from build123d import *

# Parameters (mm, degrees)
SKETCH1_R           = 1.75
BOSS_EXTRUDE1_DEPTH = 2.5
CUT_EXTRUDE1_DEPTH  = 0.2
SKETCH5_R           = 3
CUT_EXTRUDE2_DEPTH  = 0.5
CHAMFER2_SIZE       = 1


with BuildPart() as part:
    # Sketch1 → Boss-Extrude1 (new body)
    with BuildSketch(Plane.XY):
        with BuildLine():
            ThreePointArc((-28.95, 27.5), (-33.45, 23), (-28.95, 18.5))
            Line((-28.95, 18.5), (-24.45, 18.5))
            Line((-24.45, 18.5), (-24.45, -18.5))
            Line((-24.45, -18.5), (-28.95, -18.5))
            ThreePointArc((-28.95, -18.5), (-33.45, -23), (-28.95, -27.5))
            Line((-28.95, -27.5), (28.95, -27.5))
            ThreePointArc((28.95, -27.5), (33.45, -23), (28.95, -18.5))
            Line((28.95, -18.5), (24.45, -18.5))
            Line((24.45, -18.5), (24.45, 18.5))
            Line((24.45, 18.5), (28.95, 18.5))
            ThreePointArc((28.95, 18.5), (33.45, 23), (28.95, 27.5))
            Line((28.95, 27.5), (-28.95, 27.5))
        make_face()
        with Locations((-28.95, -23)):
            Circle(SKETCH1_R, mode=Mode.SUBTRACT)
        with Locations((-28.95, 23)):
            Circle(SKETCH1_R, mode=Mode.SUBTRACT)
        with Locations((28.95, 23)):
            Circle(SKETCH1_R, mode=Mode.SUBTRACT)
        with Locations((28.95, -23)):
            Circle(SKETCH1_R, mode=Mode.SUBTRACT)
    extrude(amount=BOSS_EXTRUDE1_DEPTH)

    # Sketch4 → Cut-Extrude1 (cut)
    with BuildSketch(Plane.XY.offset(2.5)):
        with BuildLine():
            Line((-6.923076923, -4.414458023), (-8.846153846, -4.414458023))
            Line((-8.846153846, -4.414458023), (-8.846153846, 2.704933003))
            add(Edge.make_bspline(
                [(-8.846153846, 2.704933003), (-8.933318023, 2.616445103), (-9.106463901, 2.440669737), (-9.383005145, 2.19548654), (-9.670097117, 1.967401521), (-9.970580856, 1.758581072), (-10.280528273, 1.566049869), (-10.603106853, 1.391327059), (-10.935978437, 1.231995104), (-11.166572995, 1.142953291), (-11.282051282, 1.09836249)],
                knots=[0, 0, 0, 0, 0.000372537, 0.00074002, 0.001107934, 0.001471928, 0.001837155, 0.002201986, 0.002572064, 0.002943306, 0.002943306, 0.002943306, 0.002943306], degree=3))
            Line((-11.282051282, 1.09836249), (-11.282051282, 3.021439413))
            add(Edge.make_bspline(
                [(-11.282051282, 3.021439413), (-11.153980048, 3.06946063), (-10.88593692, 3.1699653), (-10.490395403, 3.38374383), (-10.077539391, 3.648423218), (-9.730716774, 3.908012402), (-9.455353873, 4.138807932), (-9.26289614, 4.324331325), (-9.084572984, 4.514316902), (-8.927087219, 4.714896702), (-8.786304768, 4.922015444), (-8.661565378, 5.135334763), (-8.551766041, 5.355528522), (-8.494286856, 5.508866571), (-8.465544872, 5.585541977)],
                knots=[0, 0, 0, 0, 0.000409928, 0.000857948, 0.001345291, 0.001880548, 0.002156279, 0.002422637, 0.002682042, 0.002937331, 0.003186801, 0.003432796, 0.003678268, 0.003923781, 0.003923781, 0.003923781, 0.003923781], degree=3))
            Line((-8.465544872, 5.585541977), (-6.923076923, 5.585541977))
            Line((-6.923076923, 5.585541977), (-6.923076923, -4.414458023))
        make_face()
        with BuildLine():
            Line((2.435897436, -2.4913811), (2.435897436, -4.414458023))
            Line((2.435897436, -4.414458023), (-4.102564103, -4.414458023))
            add(Edge.make_bspline(
                [(-4.102564103, -4.414458023), (-4.080426387, -4.250103198), (-4.036163368, -3.921485704), (-3.899317938, -3.441458257), (-3.716676165, -2.973033485), (-3.518453211, -2.59184942), (-3.321298527, -2.285009365), (-3.142420071, -2.033582253), (-2.929024642, -1.766074598), (-2.684208836, -1.480326872), (-2.409325608, -1.175445832), (-2.102324151, -0.852564961), (-1.761740021, -0.513229981), (-1.522133018, -0.282804832), (-1.398237179, -0.163656741)],
                knots=[0, 0, 0, 0, 0.000496964, 0.00099365, 0.001492867, 0.002003586, 0.002279214, 0.0025866, 0.002928861, 0.003305405, 0.003715318, 0.004160237, 0.004641841, 0.005157509, 0.005157509, 0.005157509, 0.005157509], degree=3))
            add(Edge.make_bspline(
                [(-1.398237179, -0.163656741), (-1.299366883, -0.068219837), (-1.111146958, 0.113463921), (-0.843121421, 0.373627698), (-0.607499354, 0.612792158), (-0.399354228, 0.824759525), (-0.22349449, 1.014927025), (-0.077606865, 1.180308106), (0.040156295, 1.321576252), (0.103936924, 1.411196852), (0.132211538, 1.450926592)],
                knots=[0, 0, 0, 0, 0.000412257, 0.000784815, 0.001120524, 0.001419431, 0.001676006, 0.00189743, 0.002081082, 0.002227329, 0.002227329, 0.002227329, 0.002227329], degree=3))
            add(Edge.make_bspline(
                [(0.132211538, 1.450926592), (0.190111047, 1.547103861), (0.30179249, 1.73261867), (0.424260458, 2.024344061), (0.497770298, 2.316009192), (0.507857836, 2.510898163), (0.512820513, 2.606775951)],
                knots=[0, 0, 0, 0, 0.000336425, 0.000648925, 0.000945785, 0.00123325, 0.00123325, 0.00123325, 0.00123325], degree=3))
            add(Edge.make_bspline(
                [(0.512820513, 2.606775951), (0.509218846, 2.70654968), (0.502404775, 2.895313794), (0.445267605, 3.161694863), (0.343944107, 3.390687129), (0.204440295, 3.582993487), (0.028037447, 3.733664782), (-0.178182613, 3.844996243), (-0.417238616, 3.906548032), (-0.585261277, 3.914644013), (-0.673076923, 3.91887531)],
                knots=[0, 0, 0, 0, 0.000299149, 0.000565967, 0.000811668, 0.001045254, 0.001272527, 0.001501953, 0.00174248, 0.002005823, 0.002005823, 0.002005823, 0.002005823], degree=3))
            add(Edge.make_bspline(
                [(-0.673076923, 3.91887531), (-0.760299295, 3.914923595), (-0.928794085, 3.907289734), (-1.168261741, 3.840601371), (-1.377751743, 3.7251568), (-1.52704546, 3.593596575), (-1.627900447, 3.465663812), (-1.696619517, 3.354178836), (-1.755849991, 3.227497715), (-1.808333132, 3.087046666), (-1.84978888, 2.931216675), (-1.883174765, 2.761194545), (-1.910078959, 2.576065314), (-1.918634967, 2.447276207), (-1.923076923, 2.380413772)],
                knots=[0, 0, 0, 0, 0.000261347, 0.000504866, 0.000737962, 0.000973524, 0.001096162, 0.001225691, 0.001365471, 0.001515056, 0.001674936, 0.001848581, 0.002034706, 0.002235667, 0.002235667, 0.002235667, 0.002235667], degree=3))
            Line((-1.923076923, 2.380413772), (-3.846153846, 2.568715054))
            add(Edge.make_bspline(
                [(-3.846153846, 2.568715054), (-3.830692606, 2.698546985), (-3.80071573, 2.950270356), (-3.725907936, 3.311831909), (-3.631166636, 3.645388763), (-3.511975194, 3.950321896), (-3.373259936, 4.228570387), (-3.207945231, 4.475958944), (-3.021807349, 4.695227932), (-2.814685425, 4.886260652), (-2.5878962, 5.049664829), (-2.349921603, 5.195528131), (-2.096110944, 5.315182407), (-1.829258686, 5.413795508), (-1.549485425, 5.49260631), (-1.255497172, 5.544714943), (-0.949108314, 5.581368356), (-0.739966, 5.584129802), (-0.633012821, 5.585541977)],
                knots=[0, 0, 0, 0, 0.000392096, 0.000760212, 0.001106367, 0.001431121, 0.001741094, 0.002037223, 0.002321424, 0.002602116, 0.002880179, 0.003158798, 0.003438358, 0.003720412, 0.004011539, 0.004308966, 0.004615352, 0.004936021, 0.004936021, 0.004936021, 0.004936021], degree=3))
            add(Edge.make_bspline(
                [(-0.633012821, 5.585541977), (-0.516740897, 5.583307291), (-0.290286727, 5.57895496), (0.040296159, 5.543013371), (0.350855029, 5.480344005), (0.644105005, 5.397329559), (0.917034567, 5.286499204), (1.171918028, 5.152509913), (1.404743968, 4.990276522), (1.618982973, 4.808646307), (1.810495503, 4.608911963), (1.978243149, 4.395861516), (2.118781575, 4.169643399), (2.236714897, 3.93301496), (2.324279592, 3.682168505), (2.388083037, 3.420572552), (2.43038729, 3.147006702), (2.434040407, 2.960167431), (2.435897436, 2.865189413)],
                knots=[0, 0, 0, 0, 0.000348765, 0.000679263, 0.000995909, 0.001298314, 0.001592185, 0.001878054, 0.002160328, 0.002441705, 0.002719393, 0.002989083, 0.003253658, 0.003517047, 0.003780619, 0.004048809, 0.004324175, 0.004608884, 0.004608884, 0.004608884, 0.004608884], degree=3))
            add(Edge.make_bspline(
                [(2.435897436, 2.865189413), (2.433450826, 2.756184824), (2.428597126, 2.539936446), (2.382126554, 2.220256739), (2.311128567, 1.907948806), (2.206199134, 1.602249395), (2.073192931, 1.295825486), (1.901744746, 0.987989283), (1.702680436, 0.669456993), (1.546820928, 0.463511968), (1.466346154, 0.357176592)],
                knots=[0, 0, 0, 0, 0.000326823, 0.000648367, 0.000967129, 0.0012864, 0.001616516, 0.001967917, 0.002342489, 0.002742354, 0.002742354, 0.002742354, 0.002742354], degree=3))
            add(Edge.make_bspline(
                [(1.466346154, 0.357176592), (1.435930222, 0.318867637), (1.370786347, 0.236818733), (1.259959496, 0.111009427), (1.131520709, -0.026413994), (0.987284126, -0.178023781), (0.82248533, -0.338451015), (0.643053791, -0.51440464), (0.441093999, -0.696884043), (0.231912595, -0.890441198), (0.021821946, -1.078827655), (-0.171281651, -1.257753025), (-0.34668397, -1.416063548), (-0.496216198, -1.562498691), (-0.628673782, -1.687064362), (-0.739282513, -1.796148144), (-0.830112141, -1.887109206), (-0.955269523, -2.028894425), (-1.114518089, -2.220658992), (-1.226555966, -2.40389546), (-1.280048077, -2.4913811)],
                knots=[0, 0, 0, 0, 0.000146727, 0.000314255, 0.00050278, 0.000711046, 0.000941937, 0.00119269, 0.00146489, 0.001758378, 0.002047687, 0.002311396, 0.002548156, 0.002756422, 0.002939197, 0.0030936, 0.003222507, 0.003324651, 0.003660963, 0.003968244, 0.003968244, 0.003968244, 0.003968244], degree=3))
            Line((-1.280048077, -2.4913811), (2.435897436, -2.4913811))
        make_face()
        Polygon((6.774839744, -4.414458023), (3.076923077, 5.585541977), (5.108173077, 5.585541977), (7.756410256, -1.850355459), (10.39463141, 5.585541977), (12.435897436, 5.585541977), (8.752003205, -4.414458023), align=None)
    extrude(amount=-CUT_EXTRUDE1_DEPTH, mode=Mode.SUBTRACT)

    # Sketch5 → Cut-Extrude2 (cut)
    with BuildSketch(Plane.XY.offset(2.5)):
        with Locations((-28.95, 23)):
            Circle(SKETCH5_R)
        with Locations((28.95, 23)):
            Circle(SKETCH5_R)
        with Locations((28.95, -23)):
            Circle(SKETCH5_R)
        with Locations((-28.95, -23)):
            Circle(SKETCH5_R)
    extrude(amount=-CUT_EXTRUDE2_DEPTH, mode=Mode.SUBTRACT)

    # Chamfer2
    chamfer2_edges = [part.edges().sort_by_distance(p)[0] for p in [
        (-30.7, 23, 2),
        (27.2, 23, 2),
        (27.2, -23, 2),
        (-30.7, -23, 2),
    ]]
    chamfer(chamfer2_edges, length=CHAMFER2_SIZE)


solid = part.part
CAD build for the part. Positions are in the model's coordinates, mm. A direction names the side the tool comes from. Round coordinates to 2 decimals unless told otherwise and drop trailing zeros. Write each loop counter-clockwise with the first axis right and the second up, starting at its lowest first coordinate (ties: lowest second). Pieces come first, ordered by that corner, then holes. Notation, with made-up numbers: M 63.25,2 L 77.25,2 A17 ccw 77.25,13 Z; hole C -18.5,35.5 d1. An arc over 180 degrees is marked long. Use a Markdown table: item, result. Add a question column.
1. Flat gauge pins, fed straight in: P1, Ø1.8, axis at x = -28.5, y = -21.5, coming from the +Z side; P2, Ø1.5, axis at y = 22, z = 2, coming from the -X side; P3, Ø1.2, axis at y = -3, z = 0.5, coming from the +X side. Where does each tip first touch, or does it go through?
2. Drill centre lines: probe 1 along Y at (x, z) = (28.95, 0.5); probe 2 along Y at (x, z) = (-28.95, 2.4); probe 3 along Y at (x, z) = (26, 1.2). Where is each one in solid material? Low to high.
3. Pull direction Y, two halves, no side cores. Call faces 4 (the face through (0, 27.5, 1)), 5 (the face through (-33.45, -22.9, 1.23)), 6 (the face through (0, -27.5, 1)): released by +Y, released by -Y, zero draft, split by the parting line, or undercut.
4. Slice it at B-B on y = -6.5. Give the cut face in (x, z).
5. 3-axis set-ups, long thin cutter, end or side, ignore diameter. For faces 1 (the face through (-24.45, 0, 1)), 2 (the face through (27, -18.5, 1)), 3 (the face through (-31.947, 23.132, 2.254)): which of +Z, -Z, +X, -X, +Y, -Y reach the whole face in a straight line?
6. Slice it at A-A on y = 23. Give the cut face in (x, z), then the cut area to 3 significant figures.
Reply:
| question | item | result |
|---|---|---|
| 1 | P1 | stops at z = 1.72 |
| 1 | P2 | stops at x = -33.44 |
| 1 | P3 | stops at x = 24.45 |
| 2 | probe 1 | y = -27.5 to -24.75, -21.25 to -18.5, 18.5 to 21.25, 24.75 to 27.5 |
| 2 | probe 2 | y = -27.5 to -26, -20 to -18.5, 18.5 to 20, 26 to 27.5 |
| 2 | probe 3 | y = -27.5 to -18.5, 18.5 to 27.5 |
| 3 | face 4 | released by +Y |
| 3 | face 5 | undercut |
| 3 | face 6 | released by -Y |
| 4 | outline | M -24.45,0 L 24.45,0 L 24.45,2.5 L -24.45,2.5 Z |
| 5 | face 1 | +Z, -Z, -X |
| 5 | face 2 | +Z, -Z, +X |
| 5 | face 3 | +Z |
| 6 | outline | M -33.45,0 L -30.7,0 L -30.7,1 L -31.7,2 L -31.95,2 L -31.95,2.5 L -33.45,2.5 Z; M -27.2,0 L 27.2,0 L 27.2,1 L 26.2,2 L 25.95,2 L 25.95,2.5 L -25.95,2.5 L -25.95,2 L -26.2,2 L -27.2,1 Z; M 30.7,0 L 33.45,0 L 33.45,2.5 L 31.95,2.5 L 31.95,2 L 31.7,2 L 30.7,1 Z |
| 6 | area | 145 mm^2 |
